from build123d import *

# Parameters (mm, degrees)
F0_W     = 135
F0_H     = 95
F1_DEPTH = 10
F3_DEPTH = 10
F4_W     = 135
F4_H     = 5
F5_DEPTH = 5


with BuildPart() as f1:
    # F0 (on Front) → F1 (new body)
    with BuildSketch(Plane.XZ):
        with Locations((-0.448078, 7.457405)):
            Rectangle(F0_W, F0_H)
    extrude(amount=F1_DEPTH)

    # F2 (on face) → F3 (cut)
    with BuildSketch(Plane(origin=(-67.948078, 0, 0), x_dir=(0, -1, 0), z_dir=(-1, 0, 0))):
        Polygon((10, 34.957405), (0, 39.957405), (0, 19.957405), (10, 24.957405), align=None)
        Polygon((10, -10.042595), (0, -5.042595), (0, -25.042595), (10, -20.042595), align=None)
    extrude(amount=-F3_DEPTH, mode=Mode.SUBTRACT)

    # F4 (on face) → F5 (cut)
    with BuildSketch(Plane.XZ.offset(10)):
        with Locations((-0.448078, -32.542595)):
            Rectangle(F4_W, F4_H)
    extrude(amount=-F5_DEPTH, mode=Mode.SUBTRACT)

    # F6: F1 across face


with BuildPart() as f1_1:
    add(f1.part)
    add(f1.part.mirror(Plane(origin=(67.051922, -4.932432, 8.538486), x_dir=(0, 1, 0), z_dir=(1, 0, 0))))


solid = f1_1.part
Verification items for the finished model (mm, model axes). A direction names the side the tool comes from. Round coordinates to 2 decimals unless told otherwise and drop trailing zeros. Loops run counter-clockwise (first coordinate to the right, second up) from the corner with the lowest first, then second, coordinate; pieces in that order, holes last. Notation, with made-up numbers: (29, -12) - (81, -12) arc R9 cw to (81, -7) - close; hole circle Ø6 at (63, 86). An arc over 180 degrees is marked (long way). Use a Markdown table: item, result. Add a question column.
1. Access from +Z, -Z, +X, -X, +Y, -Y to the whole of each face (thin tool, end or side, straight path). Record for faces 1 (the face through (-57.948, -4, -15)), 2 (the face through (-67.948, -5, 7)), 3 (the face through (197.122, -5.07, -7.578)), 4 (the face through (69, -5, -33)), 5 (the face through (69, -10, 13)).
2. Section check A-A, the plane y = -8.25. Record the boundary of the cut face in (x, z), plus the area to 3 significant figures.
3. Section check B-B, the plane x = 137. Record the boundary of the cut face in (y, z), plus the area to 3 significant figures.
4. Thickness scan on probe 1 along Z at (x, y) = (-11.5, -6.5); probe 2 along X at (y, z) = (-8.5, -20). Record the ranges inside material, lowest first. Write a range as [from, to].
5. Release check for a two-part mould opening along Z. For faces 6 (the face through (-57.948, -4, 30)), 7 (the face through (69, -5, -40.043)), 8 (the face through (-67.948, -4, -30)) record: released by +Z, released by -Z, zero draft, split by the parting line, or undercut.
6. Gauge pin test, flat ends, axial feed: pin 1 (5 mm diameter, centred on y = -2.5, z = 26.5, fed in from -X); pin 2 (2.5 mm diameter, centred on x = 71, z = -33.5, fed in from -Y). Record the tip position at first contact, or that the pin passes through.
7. Section check C-C, the plane z = -22.5. Record the boundary of the cut face in (x, y).
Checks:
| question | item | result |
|---|---|---|
| 1 | face 1 | -X, +Y |
| 1 | face 2 | +Z, -Z, -X, +Y, -Y |
| 1 | face 3 | +X, +Y |
| 1 | face 4 | +X, -X, -Y |
| 1 | face 5 | +Z, -Z, +X, -X, -Y |
| 2 | outline | (-67.95, -40.04) - (202.05, -40.04) - (202.05, -35.04) - (-67.95, -35.04) - close; (-67.95, -30.04) - (202.05, -30.04) - (202.05, -20.92) - (192.05, -20.92) - (192.05, -9.17) - (202.05, -9.17) - (202.05, 24.08) - (192.05, 24.08) - (192.05, 35.83) - (202.05, 35.83) - (202.05, 54.96) - (-67.95, 54.96) - (-67.95, 35.83) - (-57.95, 35.83) - (-57.95, 24.08) - (-67.95, 24.08) - (-67.95, -9.17) - (-57.95, -9.17) - (-57.95, -20.92) - (-67.95, -20.92) - close |
| 2 | area | 23,800 mm^2 |
| 3 | outline | (-10, -40.04) - (0, -40.04) - (0, 54.96) - (-10, 54.96) - (-10, -30.04) - (-5, -30.04) - (-5, -35.04) - (-10, -35.04) - close |
| 3 | area | 925 mm^2 |
| 4 | probe 1 | z = [-40.04, -35.04], [-30.04, 54.96] |
| 4 | probe 2 | x = [-57.95, 192.05] |
| 5 | face 6 | undercut |
| 5 | face 7 | released by -Z |
| 5 | face 8 | zero draft |
| 6 | pin 1 | stops at x = -57.95 |
| 6 | pin 2 | stops at y = -5 |
| 7 | outline | (-67.95, -10) - (202.05, -10) - (202.05, -5.09) - (192.05, -5.09) - (192.05, 0) - (-57.95, 0) - (-57.95, -5.09) - (-67.95, -5.09) - close |
